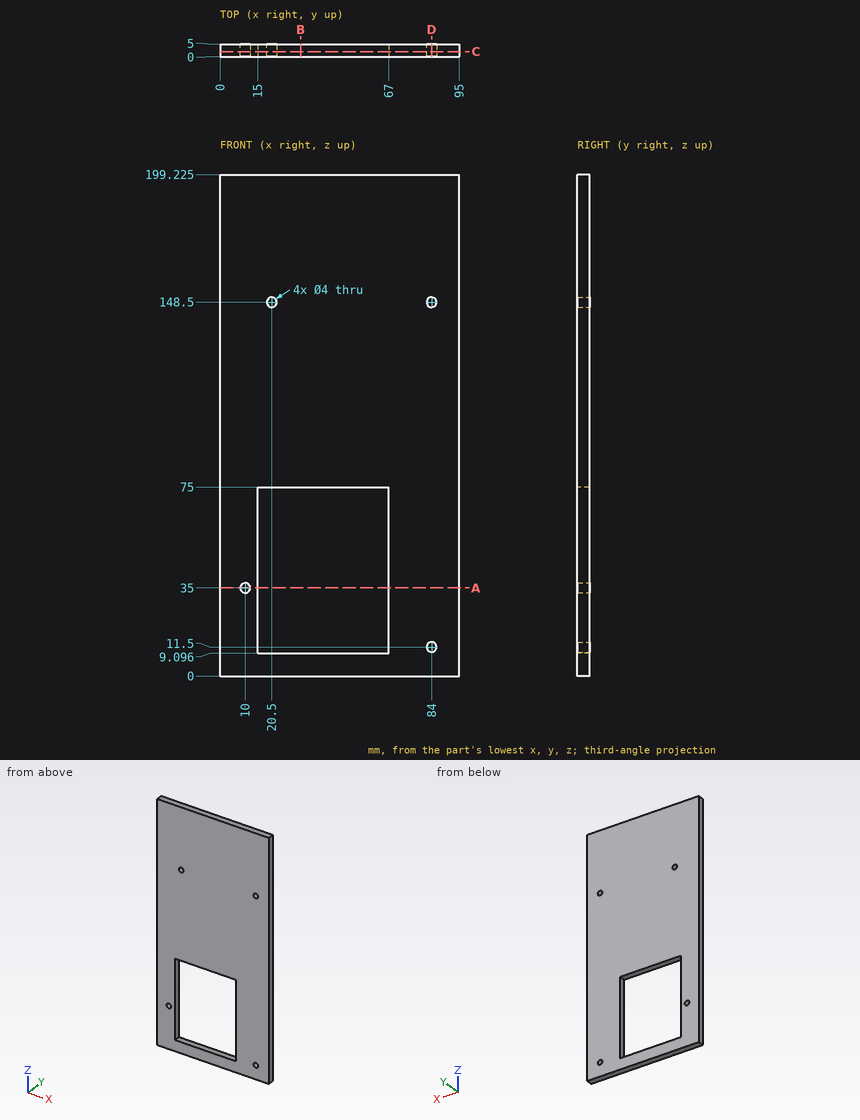
Print and shaded views of the part. All mm, measured from the part's lowest x, y and z. Coordinates: 2 decimals unless noted, no trailing zeros. Loops run counter-clockwise (first coordinate to the right, second up) from the corner with the lowest first, then second, coordinate; pieces in that order, holes last. Notation, with made-up numbers: (61.25, 37) - (96.25, 37) arc R37 ccw to (96.25, 74) - close; hole circle Ø5 at (-36.5, -22). An arc over 180 degrees is marked (long way). Use one line per item in the form item = value. Start each with the question number.
1) Band-saw the part on C-C (y = 1.95). Give the cut face in (x, z) (1 decimal), and give its area (3 significant figures).
2) Drill centre lines: L1, parallel to X at y = 2.9, z = 148.5; L2, parallel to Z at x = 84, y = 3.05 (1 decimal); L3, parallel to Z at x = 20.5, y = 1.2 (1 decimal). Where is each one in solid material? Low to high. Write a range as from..to.
3) Band-saw the part on D-D (x = 84). Give the cut face in (y, z) (1 decimal).
4) Band-saw the part on B-B (x = 32). Give the cut face in (y, z) (1 decimal).
5) Flat gauge pin, fed straight in: pin 1 (3 mm diameter, centred on x = 20.5, z = 148.5, fed in from -Y). Where does the tip first touch, or does it go through?
6) Band-saw the part on A-A (z = 35). Give the cut face in (x, y).
Check values:
q1.outline = (0, 0) - (95, 0) - (95, 199.2) - (0, 199.2) - close; hole circle Ø4 at (10, 35); hole (15, 9.1) - (67, 9.1) - (67, 75) - (15, 75) - close; hole circle Ø4 at (20.5, 148.5); hole circle Ø4 at (84, 11.5); hole circle Ø4 at (84, 148.5)
q1.area = 15,400 mm2
q2.L1 = 0..18.5, 22.5..82, 86..95
q2.L2 = 0..9.5, 13.5..146.5, 150.5..199.2
q2.L3 = 0..9.1, 75..146.5, 150.5..199.2
q3.outline = (0, 0) - (5, 0) - (5, 9.5) - (0, 9.5) - close; (0, 13.5) - (5, 13.5) - (5, 146.5) - (0, 146.5) - close; (0, 150.5) - (5, 150.5) - (5, 199.2) - (0, 199.2) - close
q4.outline = (0, 0) - (5, 0) - (5, 9.1) - (0, 9.1) - close; (0, 75) - (5, 75) - (5, 199.2) - (0, 199.2) - close
q5.pin_1 = through
q6.outline = (0, 0) - (8, 0) - (8, 5) - (0, 5) - close; (12, 0) - (15, 0) - (15, 5) - (12, 5) - close; (67, 0) - (95, 0) - (95, 5) - (67, 5) - close
